from build123d import *
from build123d.topology import SkipClean

# Parameters (mm, degrees)
SKETCH1_R               = 3.175
SKETCH1_R_2             = 2.38125
BOSS_EXTRUDE1_DEPTH     = 91.1098
CUT_EXTRUDE1_DEPTH      = 98.351934288
CUT_EXTRUDE1_DEPTH_BACK = 98.351934288
FILLET1_R               = 1.5875
BOSS_EXTRUDE2_START     = 7.3152
SKETCH3_R               = 3.175
BOSS_EXTRUDE2_DEPTH     = 7.3152
SKETCH4_R               = 2.38125
BOSS_EXTRUDE3_DEPTH     = 3.175
BOSS_EXTRUDE4_START     = -1.5875
BOSS_EXTRUDE4_DEPTH     = 1.5875


with BuildPart() as part:
    # Sketch1 → Boss-Extrude1 (new, symmetric)
    # profile 1 of 3: a face of its own
    with BuildSketch(Plane.XY):
        with BuildLine():
            Line((-33.7058, -3.175), (-33.7058, -6.35))
            Line((-33.7058, -6.35), (0, -6.35))
            Line((0, -6.35), (2.749630657, -1.5875))
            ThreePointArc((2.749630657, -1.5875), (-1.5875, -2.749630657), (-2.749630657, 1.5875))
            Line((-2.749630657, 1.5875), (-5.499261314, -3.175))
            Line((-5.499261314, -3.175), (-33.7058, -3.175))
        make_face()
    # profile 2 of 3: a face of its own
    with BuildSketch(Plane.XY):
        Circle(SKETCH1_R)
        Circle(SKETCH1_R_2, mode=Mode.SUBTRACT)
    # profile 3 of 3: a face of its own
    with BuildSketch(Plane.XY):
        Circle(SKETCH1_R_2)
    extrude(amount=BOSS_EXTRUDE1_DEPTH, both=True)

    # Sketch2 → Cut-Extrude1 (cut, two sides: drawn at the far end of the back side and taken through both)
    with BuildSketch(Plane(origin=(0, 0, 0), x_dir=(1, 0, 0), z_dir=(0, 1, 0)).offset(-CUT_EXTRUDE1_DEPTH_BACK)):
        Polygon((-5.499261314, 89.5223), (-5.499261314, -89.5223), (3.175, -89.5223), (3.175, 0), (3.175, 89.5223), align=None)
    extrude(amount=CUT_EXTRUDE1_DEPTH + CUT_EXTRUDE1_DEPTH_BACK, mode=Mode.SUBTRACT)

    # Fillet1
    fillet1_edges = [part.edges().sort_by_distance(p)[0] for p in [
        (0, -6.35, 90.31605),
        (-33.7058, -6.35, 0),
        (-33.7058, -3.175, 0),
        (-33.7058, -4.7625, 91.1098),
        (0, -6.35, -90.31605),
        (-33.7058, -4.7625, -91.1098),
    ]]
    fillet(fillet1_edges, radius=FILLET1_R - 0.0001)  # a hair under: the kernel refuses the full size

    # Sketch3 → Boss-Extrude2 (add)
    with BuildSketch(Plane.XY.offset(91.1098).offset(BOSS_EXTRUDE2_START)):
        with Locations(Location((0, 0, 0), (0, 0, 150))):
            Circle(SKETCH3_R)
    boss_extrude2 = extrude(amount=-BOSS_EXTRUDE2_DEPTH)

    # Sketch4 → Boss-Extrude3 (add)
    with BuildSketch(Plane.XY.offset(98.425)):
        Circle(SKETCH4_R)
    boss_extrude3 = extrude(amount=BOSS_EXTRUDE3_DEPTH)

    # Mirror1: Boss-Extrude2, Boss-Extrude3 across plane
    with SkipClean():  # the faces are left unmerged after this step: merging them gives an invalid solid
        add(boss_extrude2.mirror(Plane.XY))
        add(boss_extrude3.mirror(Plane.XY))

    # Sketch6 → Boss-Extrude4 (add)
    with SkipClean():  # the faces are left unmerged after this step: merging them gives an invalid solid
        with BuildSketch(Plane(origin=(0, 0, -98.425), x_dir=(-1, 0, 0), z_dir=(0, 0, -1)).offset(BOSS_EXTRUDE4_START)):
            with BuildLine():
                Line((2.749630657, 1.5875), (3.175, 0.850738686))
                Line((3.175, 0.850738686), (3.175, 25.4))
                ThreePointArc((3.175, 25.4), (0, 28.575), (-3.175, 25.4))
                Line((-3.175, 25.4), (-3.175, 0))
                ThreePointArc((-3.175, 0), (-0.821750468, 3.066814498), (2.749630657, 1.5875))
            make_face()
        boss_extrude4 = extrude(amount=BOSS_EXTRUDE4_DEPTH)

    # Mirror2: Boss-Extrude4 across plane
    with SkipClean():  # the faces are left unmerged after this step: merging them gives an invalid solid
        add(boss_extrude4.mirror(Plane.XY))


solid = part.part
The listing builds one solid part. Answer for the finished solid, in the listing's coordinates (mm). A direction names the side the tool comes from. Coordinates: 2 decimals unless noted, no trailing zeros. Loops run counter-clockwise (first coordinate to the right, second up) from the corner with the lowest first, then second, coordinate; pieces in that order, holes last. Notation, with made-up numbers: M 2.5,31 L 25.5,31 A19 cw 25.5,43 Z; hole C 55,69 d4. An arc over 180 degrees is marked long. Answer in a Markdown table with one row per item.
1) Find the intervals of material crossed by probe 1 along Y at (x, z) = (-7, -11) (3 decimals); probe 2 along Z at (x, y) = (1, 23) (1 decimal), in increasing order.
Answers below:
| item | result |
|---|---|
| probe 1 | -6.35 to -3.175 |
| probe 2 | -98.4 to -96.8, 96.8 to 98.4 |
2) Given pin 1 (8 mm diameter, centred on x = -9.5, y = 19, fed in from +Z); pin 2 (12 mm diameter, centred on x = -6.5, y = 17, fed in from +Z) (3 decimals); pin 3 (21.5 mm diameter, centred on x = -18.5, z = 31.5, fed in from +Y) (3 decimals); pin 4 (3 mm diameter, centred on x = 0, y = 15.5, fed in from -Z) (3 decimals), each flat-ended and moving along its own axis, determine where each tip first touches the part or whether it passes through.
Answers below:
| item | result |
|---|---|
| pin 1 | through |
| pin 2 | z = 98.425 |
| pin 3 | y = -3.175 |
| pin 4 | z = -98.425 |
3) Which of the six approach directions +Z, -Z, +X, -X, +Y, -Y give full straight-line access (tool end or side, diameter ignored) to faces 1 (the flat face through (-1, -2, 89.522)), 2 (the cylindrical face through (-1.89, -1.45, 99.99)), 3 (the cylindrical face through (-1.89, -1.45, -99.99)), 4 (the flat face through (0, 0, -101.6))?
Answers below:
| item | result |
|---|---|
| face 1 | +X, +Y, -Y |
| face 2 | +Z |
| face 3 | -Z |
| face 4 | -Z, +X, -X, +Y, -Y |
4) Find section A-A (y = 12). Determine the outline of the cut face in (x, z) (1 decimal).
Answers below:
| item | result |
|---|---|
| outline | M -3.2,-98.4 L 3.2,-98.4 L 3.2,-96.8 L -3.2,-96.8 Z; M -3.2,96.8 L 3.2,96.8 L 3.2,98.4 L -3.2,98.4 Z |
5) Determine the mould class of faces 5 (the flat face through (-5.499, -5, -1)), 6 (the cylindrical face through (-0.07, 28.574, 97.62)), 7 (the flat face through (0, 14, -98.425)) for opening direction Z: released by +Z, released by -Z, zero draft, split by the parting line, or undercut.
Answers below:
| item | result |
|---|---|
| face 5 | undercut |
| face 6 | zero draft |
| face 7 | released by -Z |
6) Find section C-C (x = -24). Determine the outline of the cut face in (y, z) (3 decimals).
Answers below:
| item | result |
|---|---|
| outline | M -6.35,-91.11 L -3.175,-91.11 L -3.175,91.11 L -6.35,91.11 Z |
